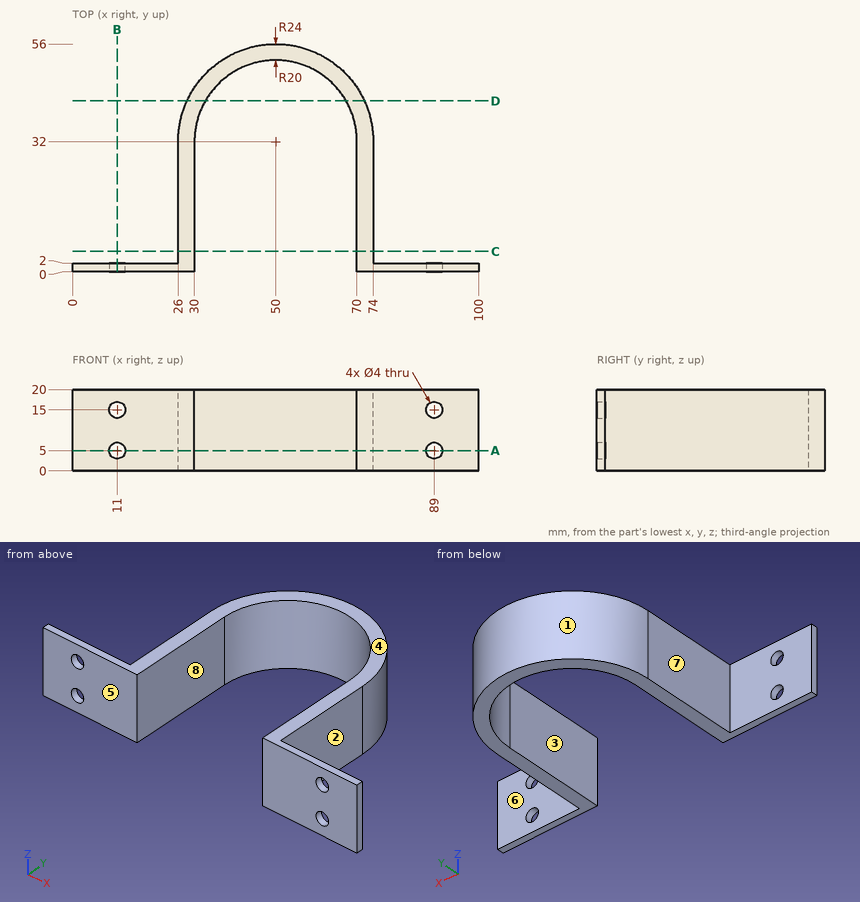
Study the drawing (mm; zero at the part's minimum x, y, z) and answer. A direction names the side the tool comes from. Round coordinates to 2 decimals unless told otherwise and drop trailing zeros. Write each loop counter-clockwise with the first axis right and the second up, starting at its lowest first coordinate (ties: lowest second). Pieces come first, ordered by that corner, then holes.
1) Determine the mould class of the marked faces 1, 2 and 3 for opening direction X: pulls with the +X half, pulls with the -X half, needs draft (parallel to the pull), parting line crosses it, or undercut.
2) Flat-ended cylindrical pins translate along their axes: P1, Ø10, axis at y = 22, z = 14.5, coming from the -X side; P2, Ø8, axis at x = 28, z = 7, coming from the +Y side; P3, Ø6.5, axis at x = 89, z = 15, coming from the -Y side; P4, Ø12, axis at y = 30.5, z = 7, coming from the +X side. Find the tip coordinate at first contact, or state that the pin passes through.
3) A cutting plane is placed at B-B on x = 11. Determine the outline of the cut face in (y, z).
4) Which of the six approach directions +Z, -Z, +X, -X, +Y, -Y give full straight-line access (tool end or side, diameter ignored) to the marked faces 4, 5, 6, 7 and 8?
5) A cutting plane is placed at C-C on y = 5. Determine the outline of the cut face in (x, z), and give its area (3 significant figures).
6) A cutting plane is placed at D-D on y = 42. Determine the outline of the cut face in (x, z), and give its area (3 significant figures).
7) Consider probe 1 along Z at (x, y) = (89, 1); probe 2 along X at (y, z) = (15, 14.75); probe 3 along Y at (x, z) = (15.5, 12.5). Determine where each line is inside the solid, lowest interval first.
8) A cutting plane is placed at A-A on z = 5. Determine the outline of the cut face in (x, y).
Entries:
1. face 1: parting line crosses it
1. face 2: pulls with the +X half
1. face 3: undercut
2. P1: stops at x = 26
2. P2: stops at y = 47.87
2. P3: stops at y = 0
2. P4: stops at x = 74
3. outline: (0, 0) - (2, 0) - (2, 3) - (0, 3) - close; (0, 7) - (2, 7) - (2, 13) - (0, 13) - close; (0, 17) - (2, 17) - (2, 20) - (0, 20) - close
4. face 4: +Z, +X, -X, +Y, -Y
4. face 5: +Z, -Z, +X, -X, -Y
4. face 6: +Z, -Z, +X, +Y
4. face 7: +Z, -Z, -X, +Y
4. face 8: +Z, -Z, -Y
5. outline: (26, 0) - (30, 0) - (30, 20) - (26, 20) - close; (70, 0) - (74, 0) - (74, 20) - (70, 20) - close
5. area: 160 mm2
6. outline: (28.18, 0) - (32.68, 0) - (32.68, 20) - (28.18, 20) - close; (67.32, 0) - (71.82, 0) - (71.82, 20) - (67.32, 20) - close
6. area: 180 mm2
7. probe 1: z = 0 to 3, 7 to 13, 17 to 20
7. probe 2: x = 26 to 30, 70 to 74
7. probe 3: y = 0 to 2
8. outline: (0, 0) - (9, 0) - (9, 2) - (0, 2) - close; (13, 0) - (30, 0) - (30, 32) arc R20 cw to (70, 32) - (70, 0) - (87, 0) - (87, 2) - (74, 2) - (74, 32) arc R24 ccw to (26, 32) - (26, 2) - (13, 2) - close; (91, 0) - (100, 0) - (100, 2) - (91, 2) - close
